The listing builds one solid part. Answer for the finished solid, in the listing's coordinates (mm). A direction names the side the tool comes from. Round coordinates to 2 decimals unless told otherwise and drop trailing zeros. Loops run counter-clockwise (first coordinate to the right, second up) from the corner with the lowest first, then second, coordinate; pieces in that order, holes last. Notation, with made-up numbers: (55.25, 27) -> (105.25, 27) arc R26 cw to (105.25, 42) -> close; hole circle Ø5 at (46.25, -35.5). An arc over 180 degrees is marked (long way). Write each question's results on one line, items separated by ' | '. Start each with the question number.
(1) The part is cut by section A-A (y = -31.5). Determine the outline of the cut face in (x, z).
(2) For faces 1 (the face through (0, -21.8, -7.5)), 2 (the face through (0, -30, -10.5)), 3 (the face through (30, -1, 0)), 4 (the face through (0.18, -4.99, -7.34)), 5 (the face through (0, -28, -12.5)), determine the directions among +Z, -Z, +X, -X, +Y, -Y from which every point of the face is accessible in a straight line to the end or side of a thin tool.
(3) The part is cut by section B-B (z = 7.5). Determine the outline of the cut face in (x, y), plus the area to 3 significant figures.
(4) Straight lines are drawn through the part: probe 1 along Y at (x, z) = (0, -8.95); probe 2 along Y at (x, z) = (0, -9.1); probe 3 along Z at (x, y) = (2, -35). For each, find the intervals that lie inside material, in ascending order.
(5) The part is cut by section C-C (x = 4). Determine the outline of the cut face in (y, z).
(6) Flat-ended cylindrical pins translate along their axes: pin 1 (2 mm diameter, centred on x = 13.5, z = 0, fed in from -Y); pin 2 (5 mm diameter, centred on x = 4, y = -32.5, fed in from +Z); pin 3 (12 mm diameter, centred on x = -2.5, y = -13.5, fed in from +Z). Find the tip coordinate at first contact, or state that the pin passes through.
(7) The part is cut by section D-D (y = -18). Determine the outline of the cut face in (x, z), plus the area to 3 significant figures.
```python
from build123d import *

# Parameters (mm, degrees)
F0_W     = 60
F0_H     = 25
F1_DEPTH = 2
F3_DEPTH = 12.5
F4_R     = 12.49999
F5_R     = 10
F5_R_2   = 8
F6_DEPTH = 3


# Not quite as in the source:
# - a fillet or chamfer is up to 0.001 mm smaller than in the source, because OpenCascade refuses the exact size


with BuildPart() as f1:
    # F0 (on Front) → F1 (new body)
    with BuildSketch(Plane.XZ):
        with Locations((17.5, 12.5)):
            Rectangle(F0_W, F0_H)
    extrude(amount=F1_DEPTH)

    # F2 (on Right) → F3 (join, symmetric)
    with BuildSketch(Plane.YZ):
        with BuildLine():
            Line((-42.5, -12.5), (-12.5, -12.5))
            ThreePointArc((-12.5, -12.5), (-3.6611652352, -8.8388347648), (0, 0))
            Line((0, 0), (-2, 0))
            ThreePointArc((-2, 0), (-5.0753787975, -7.4246212025), (-12.5, -10.5))
            Line((-12.5, -10.5), (-42.5, -10.5))
            Line((-42.5, -10.5), (-42.5, -12.5))
        make_face()
    extrude(amount=F3_DEPTH, both=True)

    # F4 (radius 12.5 in the source; OpenCascade refuses exactly that, so slightly less here)
    f4_edges = [f1.edges().sort_by_distance(p)[0] for p in [
        (-12.5, -42.5, -11.5),
        (12.5, -42.5, -11.5),
    ]]
    fillet(f4_edges, radius=F4_R)

    # F5 (on face) → F6 (join)
    with BuildSketch(Plane.XY.offset(-10.5)):
        with Locations((0, -30)):
            Circle(F5_R)
        with Locations((0, -30)):
            Circle(F5_R_2, mode=Mode.SUBTRACT)
    extrude(amount=F6_DEPTH)


solid = f1.part
```
Checked values:
1) outline: (-12.41, -12.5) -> (12.41, -12.5) -> (12.41, -10.5) -> (9.89, -10.5) -> (9.89, -7.5) -> (7.86, -7.5) -> (7.86, -10.5) -> (-7.86, -10.5) -> (-7.86, -7.5) -> (-9.89, -7.5) -> (-9.89, -10.5) -> (-12.41, -10.5) -> close
2) face 1: +Z, +X, -X, -Y | face 2: +Z | face 3: -Z, +X, +Y, -Y | face 4: +Z, +X, -X | face 5: -Z, +X, -X, +Y, -Y
3) outline: (-12.5, -2) -> (47.5, -2) -> (47.5, 0) -> (-12.5, 0) -> close | area: 120 mm2
4) probe 1: y = -40 to -38, -22 to -20, -7.01 to -3.77 | probe 2: y = -40 to -38, -22 to -20, -7.26 to -3.93 | probe 3: z = -12.5 to -10.5
5) outline: (-41.84, -12.5) -> (-12.5, -12.5) arc R12.5 ccw to (0, 0) -> (0, 25) -> (-2, 25) -> (-2, 0) arc R10.5 cw to (-12.5, -10.5) -> (-20.83, -10.5) -> (-20.83, -7.5) -> (-23.07, -7.5) -> (-23.07, -10.5) -> (-36.93, -10.5) -> (-36.93, -7.5) -> (-39.17, -7.5) -> (-39.17, -10.5) -> (-41.84, -10.5) -> close
6) pin 1: stops at y = -2 | pin 2: stops at z = -10.5 | pin 3: stops at z = -9.23
7) outline: (-12.5, -12.5) -> (12.5, -12.5) -> (12.5, -10.5) -> (-12.5, -10.5) -> close | area: 50.0 mm2
